Source: three-view drawing plus pictorial views. Frame: mm from the lowest corner of the part. Give positions to 0.01 mm unless a question says otherwise; leave off trailing zeros. Order: outer loops, then holes, each group sorted by start corner. A loop starts at its lowest first (then second) coordinate and runs counter-clockwise, first axis right, second up. Notation, with made-up numbers: (17.5, -37.75) - (44.5, -37.75) arc R17 cw to (44.5, -6.75) - close; hole circle Ø10 at (64, -9). An arc over 180 degrees is marked (long way). Use one line per item in the form item = value.
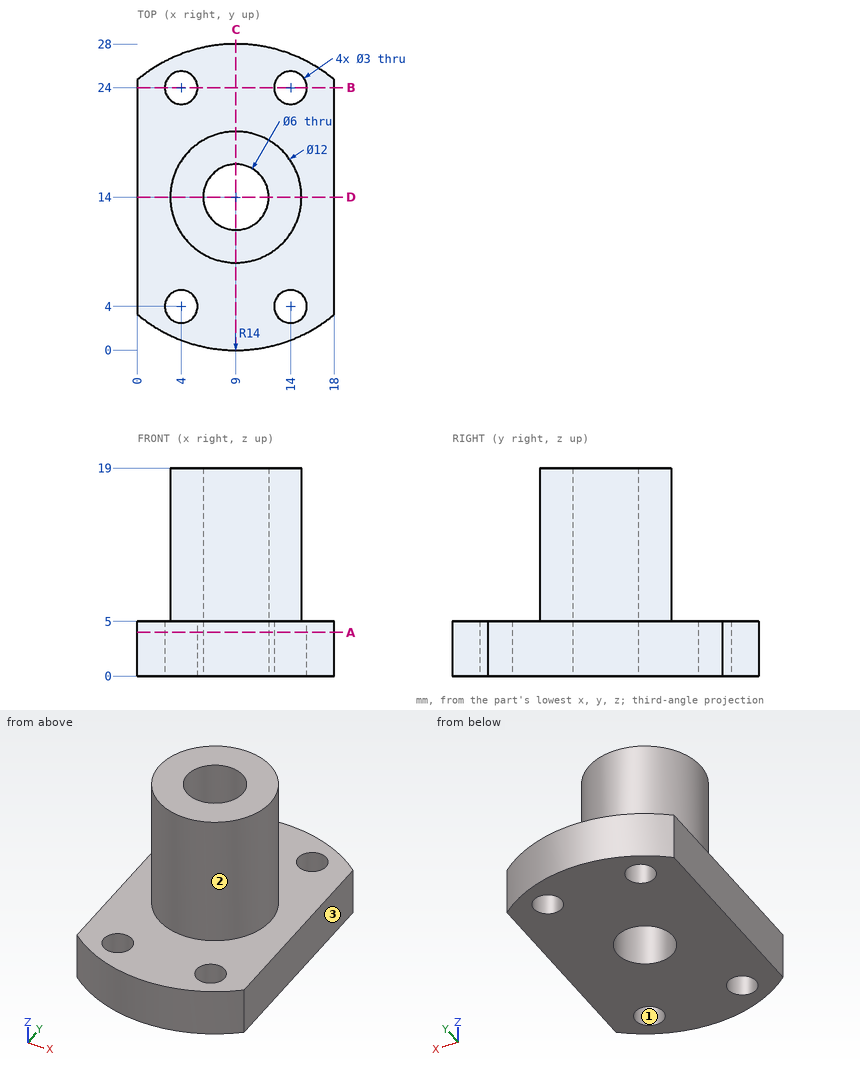
(1) Cut plane A-A on z = 4. Output: boundary loops of the cut face in (x, y).
Computed values:
outline = (0, 3.28) arc R14 ccw to (18, 3.28) - (18, 24.72) arc R14 ccw to (0, 24.72) - close; hole circle Ø3 at (4, 4); hole circle Ø3 at (4, 24); hole circle Ø6 at (9, 14); hole circle Ø3 at (14, 4); hole circle Ø3 at (14, 24)
(2) Cut plane C-C on x = 9. Output: boundary loops of the cut face in (y, z).
Computed values:
outline = (0, 0) - (11, 0) - (11, 19) - (8, 19) - (8, 5) - (0, 5) - close; (17, 0) - (28, 0) - (28, 5) - (20, 5) - (20, 19) - (17, 19) - close
(3) Cut plane D-D on y = 14. Output: boundary loops of the cut face in (x, z).
Computed values:
outline = (0, 0) - (6, 0) - (6, 19) - (3, 19) - (3, 5) - (0, 5) - close; (12, 0) - (18, 0) - (18, 5) - (15, 5) - (15, 19) - (12, 19) - close
(4) Pull-direction query (X, two-part tool) for the marked faces 1, 2 and 3; classes: released by +X, released by -X, zero draft, split by the parting line, or undercut.
Computed values:
face_1 = undercut
face_2 = split by the parting line
face_3 = released by +X
(5) Ray query, line 1 along Y through (x, z) = (14, 2.45); line 2 along Z through (x, y) = (4.5, 6.5); line 3 along Y through (x, z) = (13, 3.5). Return the intervals inside material, ascending.
Computed values:
line_1 = 0.92 to 2.5, 5.5 to 22.5, 25.5 to 27.08
line_2 = 0 to 5
line_3 = 0.58 to 2.88, 5.12 to 22.88, 25.12 to 27.42
(6) Cut plane B-B on y = 24. Output: boundary loops of the cut face in (x, z), plus the area to 3 significant figures.
Computed values:
outline = (0, 0) - (2.5, 0) - (2.5, 5) - (0, 5) - close; (5.5, 0) - (12.5, 0) - (12.5, 5) - (5.5, 5) - close; (15.5, 0) - (18, 0) - (18, 5) - (15.5, 5) - close
area = 60.0 mm²
(7) Contact query for flat-ended pins moving along their axis: pin 1 Ø4 at (x, y) = (4, 4) entering from +Z; pin 2 Ø1 at (y, z) = (15, 6.5) entering from +X; pin 3 Ø5 at (x, z) = (5, 2) entering from -Y. Output: stop coordinate, or through.
Computed values:
pin_1 = 5
pin_2 = 14.98
pin_3 = 0.08
